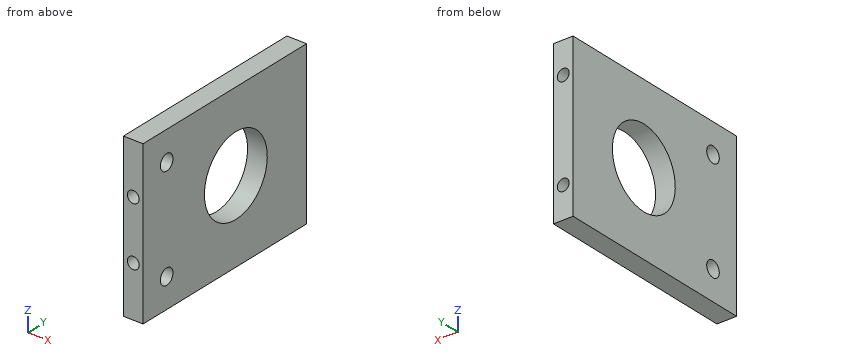
from build123d import *

# Parameters (mm, degrees)
SKETCH1_W           = 41
SKETCH1_H           = 52
SKETCH1_R           = 2
SKETCH1_R_2         = 10
BOSS_EXTRUDE1_DEPTH = 5
SKETCH2_R           = 1.5
CUT_EXTRUDE1_DEPTH  = 7
SKETCH3_R           = 1.5
CUT_EXTRUDE2_DEPTH  = 7


with BuildPart() as part:
    # Sketch1 → Boss-Extrude1 (new body)
    with BuildSketch(Plane(origin=(0, 0, 0), x_dir=(0, 0, -1), z_dir=(1, 0, 0))):
        with Locations((20.5, 26)):
            Rectangle(SKETCH1_W, SKETCH1_H)
        with Locations((7.5, 7.5)):
            Circle(SKETCH1_R, mode=Mode.SUBTRACT)
        with Locations((33.5, 7.5)):
            Circle(SKETCH1_R, mode=Mode.SUBTRACT)
        with Locations((20.143024766, 29.5)):
            Circle(SKETCH1_R_2, mode=Mode.SUBTRACT)
    extrude(amount=BOSS_EXTRUDE1_DEPTH)

    # Sketch2 → Cut-Extrude1 (cut)
    with BuildSketch(Plane(origin=(0, 0, 0), x_dir=(-1, 0, 0), z_dir=(0, -1, 0))):
        with Locations(Location((-2.5, 13, 0), (0, 0, 90))):
            Circle(SKETCH2_R)
        with Locations(Location((-2.5, 28, 0), (0, 0, 90))):
            Circle(SKETCH2_R)
    extrude(amount=-CUT_EXTRUDE1_DEPTH, mode=Mode.SUBTRACT)

    # Sketch3 → Cut-Extrude2 (cut)
    with BuildSketch(Plane(origin=(0, 52, 0), x_dir=(1, 0, 0), z_dir=(0, 1, 0))):
        with Locations(Location((2.5, 8, 0), (0, 0, 270))):
            Circle(SKETCH3_R)
        with Locations(Location((2.5, 33, 0), (0, 0, 270))):
            Circle(SKETCH3_R)
    extrude(amount=-CUT_EXTRUDE2_DEPTH, mode=Mode.SUBTRACT)


solid = part.part
Verification items for the finished model (mm, model axes). Give positions to 0.01 mm unless a question says otherwise; leave off trailing zeros. Write each loop counter-clockwise with the first axis right and the second up, starting at its lowest first coordinate (ties: lowest second). Pieces come first, ordered by that corner, then holes. Notation, with made-up numbers: M 41.25,71 L 89.25,71 A28 cw 89.25,93 Z; hole C 23.25,-36.75 d10. An arc over 180 degrees is marked long. Put each result on its own line as item: value. Start each with the question number.
1. Section check C-C (z = -33.5). Record the cut outline in (x, y), and give its area (3 significant figures).
2. Scan lines: line 1 along Y through (x, z) = (4.3, -20); line 2 along Y through (x, z) = (4.6, -33.5); line 3 along X through (y, z) = (47.5, -8). Record each from-to range of solid material in increasing order. Write a range as [from, to].
3. Section check B-B (y = 26). Record the cut outline in (x, z), and give its area (3 significant figures).
4. Section check A-A (x = 2.5). Record the cut outline in (y, z).
5. Go/stop test with flat-tipped pins: pin 1 Ø2.5 at (x, z) = (2.5, -33) entering from +Y; pin 2 Ø3 at (x, y) = (3.5, 33.5) entering from +Z; pin 3 Ø0.9 at (x, z) = (2, -28) entering from -Y. Record where each tip stops, or that it passes through.
6. Section check D-D (z = -18). Record the cut outline in (x, y).
Answer list:
1. outline: M 0,0 L 5,0 L 5,5.5 L 0,5.5 Z; M 0,9.5 L 5,9.5 L 5,52 L 3.91,52 L 3.91,45 L 1.09,45 L 1.09,52 L 0,52 Z
1. area: 220 mm2
2. line 1: [0, 19.5], [39.5, 52]
2. line 2: [0, 5.5], [9.5, 52]
2. line 3: [0, 1], [4, 5]
3. outline: M 0,-41 L 5,-41 L 5,-29.51 L 0,-29.51 Z; M 0,-10.78 L 5,-10.78 L 5,0 L 0,0 Z
3. area: 111 mm2
4. outline: M 0,-41 L 52,-41 L 52,-34.5 L 45,-34.5 L 45,-31.5 L 52,-31.5 L 52,-9.5 L 45,-9.5 L 45,-6.5 L 52,-6.5 L 52,0 L 0,0 L 0,-11.5 L 7,-11.5 L 7,-14.5 L 0,-14.5 L 0,-26.5 L 7,-26.5 L 7,-29.5 L 0,-29.5 Z; hole C 7.5,-33.5 d4; hole C 7.5,-7.5 d4; hole C 29.5,-20.14 d20
5. pin 1: y = 45
5. pin 2: z = 0
5. pin 3: y = 7
6. outline: M 0,0 L 5,0 L 5,19.73 L 0,19.73 Z; M 0,39.27 L 5,39.27 L 5,52 L 0,52 Z
